Can you work these out from the model? Positions are in its coordinate system, mm. A direction names the side the tool comes from. Round coordinates to 2 decimals unless told otherwise and drop trailing zeros. Order: outer loops, then holes, each group sorted by start corner. A loop starts at its lowest first (then second) coordinate and runs counter-clockwise, first axis right, second up. Notation, with made-up numbers: (-23, 33.5) -> (-16, 33.5) arc R26 cw to (-16, 50.5) -> close; hole circle Ø9 at (69, 83). An arc over 180 degrees is marked (long way). Use a Markdown table: item, result. Add a question column.
Q1. We'd pull the mould along Z, two halves only. Please class faces 3 (the face through (19, 0, -5)), 4 (the face through (19, 5, -10)), 5 (the face through (0.5, 5.1, -5)): +Z half, -Z half, draft (parallel to the pull), parting line (faces both ways), or undercut.
Q2. I need wall thicknesses on line 1 along Z through (x, y) = (31, 7); line 2 along X through (y, z) = (7.75, -3.75); line 3 along Z through (x, y) = (29.5, 9.75). Which ranges of each line are inside material? Lowest first, please. Write a range as [from, to].
Q3. If we section it at D-D on x = 24.5: List the corners of the cut face in (y, z) for me.
Q4. If we section it at B-B on x = 5: List the corners of the cut face in (y, z) for me.
Q5. I'm going to push a flat-ended pin straight in: pin 1 Ø2 at (x, z) = (31, -2.5) entering from +Y. Where does the tip first touch, or does it pass through?
Q6. If we section it at A-A on z = -3: List the corners of the cut face in (x, y) for me, plus the area to 3 significant figures.
Q7. For faces 1 (the face through (37.5, 5.1, -5)), 2 (the face through (5, 8, -6.2)), which set-ups out of +Z, -Z, +X, -X, +Y, -Y let a thin tool reach every point of the face, with its end or its side?
Q8. If we section it at C-C on z = -5: List the corners of the cut face in (x, y) for me, plus the area to 3 significant figures.
```python
from build123d import *

# Parameters (mm, degrees)
SKETCH1_W           = 38
SKETCH1_H           = 10
BOSS_EXTRUDE1_DEPTH = 10
SKETCH3_R           = 0.5
CUT_EXTRUDE1_DEPTH  = 41.546269865
SKETCH4_W           = 5.6
SKETCH4_H           = 2.6
CUT_EXTRUDE2_DEPTH  = 4.2
CHAMFER1_SIZE       = 0.5


with BuildPart() as part:
    # Sketch1 → Boss-Extrude1 (new body)
    with BuildSketch(Plane(origin=(0, 0, 0), x_dir=(1, 0, 0), z_dir=(0, 1, 0))):
        with Locations((19, 5)):
            Rectangle(SKETCH1_W, SKETCH1_H)
    extrude(amount=BOSS_EXTRUDE1_DEPTH)

    # Sketch2 → Cut-Revolve1 (revolve, cut)
    with BuildSketch(Plane(origin=(0, 10, 0), x_dir=(1, 0, 0), z_dir=(0, 1, 0))):
        Polygon((0, 5), (38, 5), (38, 4.5), (26.25, 4.5), (26.25, 3.6), (11.75, 3.6), (11.75, 4.5), (0, 4.5), align=None)
    revolve(axis=Axis((0, 10, -5), (1, 0, 0)), mode=Mode.SUBTRACT)

    # Sketch3 → Cut-Extrude1 (cut, through all)
    with BuildSketch(Plane(origin=(0, 10, 0), x_dir=(1, 0, 0), z_dir=(0, 1, 0))):
        with Locations((0, 5)):
            Circle(SKETCH3_R)
        with Locations((38, 5)):
            Circle(SKETCH3_R)
    extrude(amount=-CUT_EXTRUDE1_DEPTH, mode=Mode.SUBTRACT)

    # Sketch4 → Cut-Extrude2 (cut)
    with BuildSketch(Plane(origin=(0, 10, 0), x_dir=(1, 0, 0), z_dir=(0, 1, 0))):
        with Locations((5.5, 7.5)):
            Rectangle(SKETCH4_W, SKETCH4_H)
        with Locations((5.5, 2.5)):
            Rectangle(SKETCH4_W, SKETCH4_H)
        with Locations((32.5, 7.5)):
            Rectangle(SKETCH4_W, SKETCH4_H)
        with Locations((32.5, 2.5)):
            Rectangle(SKETCH4_W, SKETCH4_H)
    extrude(amount=-CUT_EXTRUDE2_DEPTH, mode=Mode.SUBTRACT)

    # Chamfer1
    chamfer1_edges = [part.edges().sort_by_distance(p)[0] for p in [
        (35.3, 10, -2.5),
        (32.5, 10, -1.2),
        (29.7, 10, -2.5),
        (35.3, 10, -7.5),
        (29.7, 10, -7.5),
        (32.5, 10, -8.8),
        (8.3, 10, -2.5),
        (5.5, 10, -1.2),
        (2.7, 10, -2.5),
        (2.7, 10, -7.5),
        (5.5, 10, -8.8),
    ]]
    chamfer(chamfer1_edges, length=CHAMFER1_SIZE)


solid = part.part
```
Answer below:
| question | item | result |
|---|---|---|
| 1 | face 3 | draft |
| 1 | face 4 | -Z half |
| 1 | face 5 | undercut |
| 2 | line 1 | [-10, -8.8], [-6.2, -3.8], [-1.2, 0] |
| 2 | line 2 | [0, 2.7], [8.3, 29.7], [35.3, 38] |
| 2 | line 3 | [-10, -9.05], [-6.2, -5.43], [-4.57, -3.8], [-0.95, 0] |
| 3 | outline | (0, -10) -> (10, -10) -> (10, -6.4) arc R1.4 cw to (10, -3.6) -> (10, 0) -> (0, 0) -> close |
| 4 | outline | (0, -10) -> (10, -10) -> (10, -9.3) -> (9.5, -8.8) -> (5.8, -8.8) -> (5.8, -6.2) -> (10, -6.2) -> (10, -5.5) arc R0.5 cw to (10, -4.5) -> (10, -3.8) -> (5.8, -3.8) -> (5.8, -1.2) -> (9.5, -1.2) -> (10, -0.7) -> (10, 0) -> (0, 0) -> close |
| 5 | pin 1 | y = 5.8 |
| 6 | outline | (0, 0) -> (38, 0) -> (38, 10) -> (35.8, 10) -> (35.3, 9.5) -> (35.3, 5.8) -> (29.7, 5.8) -> (29.7, 9.5) -> (29.2, 10) -> (8.8, 10) -> (8.3, 9.5) -> (8.3, 5.8) -> (2.7, 5.8) -> (2.7, 9.5) -> (2.2, 10) -> (0, 10) -> close |
| 6 | area | 332 mm² |
| 7 | face 1 | +X, +Y, -Y |
| 7 | face 2 | +Y |
| 8 | outline | (0.5, 0) -> (37.5, 0) -> (37.5, 9.5) -> (26.25, 9.5) -> (26.25, 8.6) -> (11.75, 8.6) -> (11.75, 9.5) -> (0.5, 9.5) -> close |
| 8 | area | 338 mm² |
